Can you work these out from the model? Positions are in its coordinate system, mm. A direction names the side the tool comes from. Give positions to 0.01 mm unless a question says otherwise; leave off trailing zeros. Loops run counter-clockwise (first coordinate to the right, second up) from the corner with the lowest first, then second, coordinate; pieces in that order, holes last.
from build123d import *

# Parameters (mm, degrees)
PAD_DEPTH           = 6
PAD001_DEPTH        = 2
SKETCH002_W         = 2.8
SKETCH002_H         = 2.8
PAD002_DEPTH        = 2
LINEARPATTERN_COUNT = 5
LINEARPATTERN_PITCH = 7.5


with BuildPart() as part:
    # Sketch → Pad (new body)
    with BuildSketch(Plane.XY):
        with BuildLine():
            Line((-27.5, 4), (27.5, 4))
            ThreePointArc((27.5, -4), (31.5, 0), (27.5, 4))
            Line((27.5, -4), (-27.5, -4))
            ThreePointArc((-27.5, 4), (-31.5, 0), (-27.5, -4))
        make_face()
        with BuildLine():
            ThreePointArc((-27.5, 3.2), (-30.7, 0), (-27.5, -3.2))
            Line((-27.5, -3.2), (-21.5, -3.2))
            ThreePointArc((-21.5, -3.2), (-18.3, 0), (-21.5, 3.2))
            Line((-27.5, 3.2), (-21.5, 3.2))
        make_face(mode=Mode.SUBTRACT)
        with BuildLine():
            ThreePointArc((21.5, 3.2), (18.3, 0), (21.5, -3.2))
            Line((21.5, -3.2), (27.5, -3.2))
            ThreePointArc((27.5, -3.2), (30.7, 0), (27.5, 3.2))
            Line((21.5, 3.2), (27.5, 3.2))
        make_face(mode=Mode.SUBTRACT)
    extrude(amount=PAD_DEPTH)

    # Sketch001 → Pad001 (new body)
    with BuildSketch(Plane.XY.offset(6)):
        with BuildLine():
            ThreePointArc((-27.5, 3.5), (-31, 0), (-27.5, -3.5))
            Line((-27.5, -3.5), (-21.5, -3.5))
            ThreePointArc((-21.5, -3.5), (-18, 0), (-21.5, 3.5))
            Line((-27.5, 3.5), (-21.5, 3.5))
        make_face()
        with BuildLine():
            ThreePointArc((-27.5, 1.45), (-28.95, 0), (-27.5, -1.45))
            Line((-27.5, -1.45), (-21.5, -1.45))
            ThreePointArc((-21.5, -1.45), (-20.05, 0), (-21.5, 1.45))
            Line((-27.5, 1.45), (-21.5, 1.45))
        make_face(mode=Mode.SUBTRACT)
        with BuildLine():
            ThreePointArc((21.5, 3.5), (18, 0), (21.5, -3.5))
            Line((21.5, -3.5), (27.499981, -3.5))
            ThreePointArc((27.499981, -3.5), (31, -9e-06), (27.5, 3.5))
            Line((21.5, 3.5), (27.5, 3.5))
        make_face()
        with BuildLine():
            ThreePointArc((21.5, 1.45), (20.05, 0), (21.5, -1.45))
            Line((21.5, -1.45), (27.5, -1.45))
            ThreePointArc((27.5, -1.45), (28.95, 0), (27.5, 1.45))
            Line((21.5, 1.45), (27.5, 1.45))
        make_face(mode=Mode.SUBTRACT)
    extrude(amount=PAD001_DEPTH)

    # Sketch002 → Pad002 (new body)
    with BuildSketch(Plane.XZ.offset(4)):
        with Locations((13.6, 4.4)):
            Rectangle(SKETCH002_W, SKETCH002_H)
    pad002 = extrude(amount=PAD002_DEPTH)

    # LinearPattern: Pad002 ×5
    with Locations(*[(-i * LINEARPATTERN_PITCH, 0, 0) for i in range(1, LINEARPATTERN_COUNT)]):
        add(pad002)


solid = part.part
(1) Suppose I cut it at C-C on x = 13. List the corners of the cut face in (y, z) for me, plus the area to 3 significant figures.
Returned:
outline: (-6, 3) - (-4, 3) - (-4, 0) - (4, 0) - (4, 6) - (-4, 6) - (-4, 5.8) - (-6, 5.8) - close
area: 53.6 mm2
(2) Suppose I cut it at B-B on y = -0.75. List the corners of the cut face in (x, z) for me, plus the area to 3 significant figures.
Returned:
outline: (-31.43, 0) - (-30.61, 0) - (-30.61, 6) - (-28.74, 6) - (-28.74, 8) - (-30.92, 8) - (-30.92, 6) - (-31.43, 6) - close; (-20.26, 6) - (-18.39, 6) - (-18.39, 0) - (18.39, 0) - (18.39, 6) - (20.26, 6) - (20.26, 8) - (18.08, 8) - (18.08, 6) - (-18.08, 6) - (-18.08, 8) - (-20.26, 8) - close; (28.74, 6) - (30.61, 6) - (30.61, 0) - (31.43, 0) - (31.43, 6) - (30.92, 6) - (30.92, 8) - (28.74, 8) - close
area: 248 mm2
(3) Suppose I cut it at A-A on z = 5.25. Give the number of separate pieces and of enclosed holes in the cut face, plus the area to 3 significant figures.
Returned:
separate pieces: 1
enclosed holes: 2
area: 377 mm2
(4) Will these pins go through, and if not, where does the flat tip stop? P1, Ø0.6, axis at y = -5, z = 4.5, coming from the +X side; P2, Ø1.6, axis at x = 13.5, y = -4.5, coming from the +Z side; P3, Ø6, axis at x = -17.5, y = 1, coming from the -Z side; P4, Ø0.6, axis at x = 6.5, y = -5, coming from the -Z side.
Returned:
P1: stops at x = 15
P2: stops at z = 6
P3: stops at z = 0
P4: stops at z = 3
(5) Please list where these lines run through material, in increasing order: probe 1 along X at (y, z) = (0, 2.5); probe 2 along Y at (x, z) = (-26, 2.25); probe 3 along X at (y, z) = (-0.25, 6.5).
Returned:
probe 1: x = -31.5 to -30.7, -18.3 to 18.3, 30.7 to 31.5
probe 2: y = -4 to -3.2, 3.2 to 4
probe 3: x = -30.99 to -28.93, -20.07 to -18.01, 18.01 to 20.07, 28.93 to 30.99
(6) Thinking about a two-plate mould opening in Y: for faces 1 (the flat face through (-25, -1.45, 7)), 2 (the flat face through (-16, -5, 3)), 3 (the flat face through (-16, -6, 4)), which applies, pulls with the +Y half, pulls with the -Y half, needs draft (parallel to the pull), parting line crosses it, or undercut?
Returned:
face 1: undercut
face 2: needs draft
face 3: pulls with the -Y half
(7) Suppose I cut it at D-D on z = 1.5. List the corners of the cut face in (x, y) for me, plus the area to 3 significant figures.
Returned:
outline: (-27.5, -4) - (27.5, -4) arc R4 ccw to (27.5, 4) - (-27.5, 4) arc R4 ccw to start; hole (-27.5, -3.2) - (-21.5, -3.2) arc R3.2 ccw to (-21.5, 3.2) - (-27.5, 3.2) arc R3.2 ccw to start; hole (21.5, -3.2) - (27.5, -3.2) arc R3.2 ccw to (27.5, 3.2) - (21.5, 3.2) arc R3.2 ccw to start
area: 349 mm2
(8) Which directions (+Z, -Z, +X, -X, +Y, -Y) give clear straight access to the entire face, cutting with the end or side of a thin tool? Please do faces 4 (the cylindrical face through (-18, 0, 7)), 5 (the flat face through (0, -5, 4)), 6 (the flat face through (15, -5, 4)), 7 (the flat face through (-1, -5, 3)), 8 (the flat face through (24, -3.5, 7)).
Returned:
face 4: +Z
face 5: +Z, -Z, -Y
face 6: +Z, -Z, +X, -Y
face 7: -Z, +X, -X, -Y
face 8: +Z, +X, -X, -Y
